```python
from build123d import *

# Parameters (mm, degrees)
SKETCH_1_W      = 22
SKETCH_1_H      = 70
SKETCH_1_R      = 2
EXTRUDE_1_DEPTH = 3
FILLET_1_R      = 4


with BuildPart() as part:
    # 草图1 → 凸台-拉伸1 (new body)
    # profile 1 of 3: a face of its own
    with BuildSketch(Plane(origin=(0, 0, 0), x_dir=(1, 0, 0), z_dir=(0, 1, 0))):
        Rectangle(SKETCH_1_W, SKETCH_1_H)
    # profile 2 of 3: a face of its own
    with BuildSketch(Plane(origin=(0, 0, 0), x_dir=(1, 0, 0), z_dir=(0, 1, 0))):
        Polygon((-45, 35), (-11, 35), (11, 35), (45, 35), (45, 55), (-45, 55), align=None)
        with Locations(Location((-27.5, 45, 0), (0, 0, 270))):
            Circle(SKETCH_1_R, mode=Mode.SUBTRACT)
        with Locations(Location((0, 45, 0), (0, 0, 270))):
            Circle(SKETCH_1_R, mode=Mode.SUBTRACT)
        with Locations(Location((27.5, 45, 0), (0, 0, 270))):
            Circle(SKETCH_1_R, mode=Mode.SUBTRACT)
    # profile 3 of 3: a face of its own
    with BuildSketch(Plane(origin=(0, 0, 0), x_dir=(1, 0, 0), z_dir=(0, 1, 0))):
        Polygon((11, -35), (-11, -35), (-45, -35), (-45, -55), (45, -55), (45, -35), align=None)
        with Locations(Location((-27.5, -45, 0), (0, 0, 270))):
            Circle(SKETCH_1_R, mode=Mode.SUBTRACT)
        with Locations(Location((0, -45, 0), (0, 0, 270))):
            Circle(SKETCH_1_R, mode=Mode.SUBTRACT)
        with Locations(Location((27.5, -45, 0), (0, 0, 270))):
            Circle(SKETCH_1_R, mode=Mode.SUBTRACT)
    extrude(amount=EXTRUDE_1_DEPTH)

    # 圆角1
    fillet_1_edges = [part.edges().sort_by_distance(p)[0] for p in [
        (11, 1.5, 35),
        (45, 1.5, 35),
        (45, 1.5, 55),
        (-45, 1.5, 55),
        (-45, 1.5, 35),
        (-11, 1.5, 35),
        (-11, 1.5, -35),
        (-45, 1.5, -35),
        (-45, 1.5, -55),
        (45, 1.5, -55),
        (45, 1.5, -35),
        (11, 1.5, -35),
    ]]
    fillet(fillet_1_edges, radius=FILLET_1_R)


solid = part.part
```
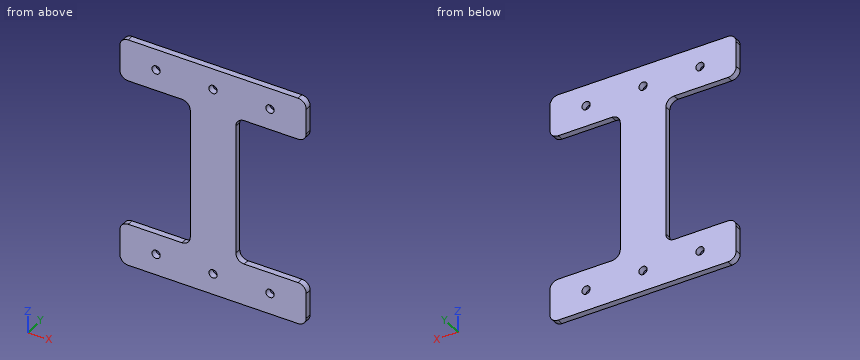
Check sheet for the modelled part. Datum: model origin and axes. Units: mm. Round coordinates to 2 decimals unless told otherwise and drop trailing zeros. Order: outer loops, then holes, each group sorted by start corner. A loop starts at its lowest first (then second) coordinate and runs counter-clockwise, first axis right, second up. Notation, with made-up numbers: (41, 21.5) - (58, 21.5) arc R21 ccw to (58, 27.5) - close; hole circle Ø5 at (46.25, 67). An arc over 180 degrees is marked (long way). Answer as CSV lines item,"result". Start each with the question number.
1) Section check A-A (x = -34.5). Record the cut outline in (y, z), then the cut area to 3 significant figures.
2) Section check B-B (y = 1.6). Give the number of separate pieces and of enclosed holes in the cut face, then the cut area to 3 significant figures.
3) Section check C-C (x = 27.5). Record the cut outline in (y, z), then the cut area to 3 significant figures.
4) Depth check by flat-ended pin: pin 1 (3.5 mm diameter, centred on x = -27.5, z = -45, fed in from +Y); pin 2 (1.5 mm diameter, centred on y = 2, z = 4.5, fed in from -X). Enter the tip coordinate at first touch or a pass-through.
5) Section check D-D (z = 45). Record the cut outline in (x, y), then the cut area to 3 significant figures.
6) Scan lines: probe 1 along X at (y, z) = (1.9, 45); probe 2 along Z at (x, y) = (23, 1.2); probe 3 along Z at (x, y) = (-1, 0.65). Record each from-to range of solid material in increasing order.
Determined:
1,outline,"(0, -55) - (3, -55) - (3, -35) - (0, -35) - close; (0, 35) - (3, 35) - (3, 55) - (0, 55) - close"
1,area,"120 mm^2"
2,separate pieces,"1"
2,enclosed holes,"6"
2,area,"5,050 mm^2"
3,outline,"(0, -55) - (3, -55) - (3, -47) - (0, -47) - close; (0, -43) - (3, -43) - (3, -35) - (0, -35) - close; (0, 35) - (3, 35) - (3, 43) - (0, 43) - close; (0, 47) - (3, 47) - (3, 55) - (0, 55) - close"
3,area,"96.0 mm^2"
4,pin 1,"through"
4,pin 2,"x = -11"
5,outline,"(-45, 0) - (-29.5, 0) - (-29.5, 3) - (-45, 3) - close; (-25.5, 0) - (-2, 0) - (-2, 3) - (-25.5, 3) - close; (2, 0) - (25.5, 0) - (25.5, 3) - (2, 3) - close; (29.5, 0) - (45, 0) - (45, 3) - (29.5, 3) - close"
5,area,"234 mm^2"
6,probe 1,"-45 to -29.5, -25.5 to -2, 2 to 25.5, 29.5 to 45"
6,probe 2,"-55 to -35, 35 to 55"
6,probe 3,"-55 to -46.73, -43.27 to 43.27, 46.73 to 55"
